```python
from build123d import *

# Parameters (mm, degrees)
SKETCH1_W                 = 270
SKETCH1_H                 = 130
SKETCH1_W_2               = 246
SKETCH1_H_2               = 106
BOSS_EXTRUDE1_DEPTH       = 12
SKETCH3_R                 = 2
CUT_EXTRUDE1_DEPTH        = 50.25
LPATTERN1_COUNT           = 2
LPATTERN1_PITCH           = 31
LPATTERN1_COPY_1_SKETCH_R = 2
LPATTERN1_COPY_1_DEPTH    = 50.25
LPATTERN2_COUNT           = 2
LPATTERN2_PITCH           = 161
MIRROR2_COPY_1_SKETCH_R   = 2
MIRROR2_COPY_1_DEPTH      = 50.25
MIRROR2_COPY_2_SKETCH_R   = 2
MIRROR2_COPY_2_DEPTH      = 50.25


with BuildPart() as part:
    # Sketch1 → Boss-Extrude1 (new body)
    with BuildSketch(Plane(origin=(0, 0, 0), x_dir=(1, 0, 0), z_dir=(0, 1, 0))):
        Rectangle(SKETCH1_W, SKETCH1_H)
        Rectangle(SKETCH1_W_2, SKETCH1_H_2, mode=Mode.SUBTRACT)
    extrude(amount=BOSS_EXTRUDE1_DEPTH)

    # Sketch3 → Cut-Extrude1 (cut)
    with BuildSketch(Plane(origin=(0, 12, 0), x_dir=(1, 0, 0), z_dir=(0, 1, 0))):
        with Locations((-65.5, -59)):
            Circle(SKETCH3_R)
    cut_extrude1 = extrude(amount=-CUT_EXTRUDE1_DEPTH, mode=Mode.SUBTRACT)

    # Mirror1: Cut-Extrude1 across plane
    add(cut_extrude1.mirror(Plane.XY), mode=Mode.SUBTRACT)

    # LPattern1: Cut-Extrude1 ×2
    with Locations(*[(i * LPATTERN1_PITCH, 0, 0) for i in range(1, LPATTERN1_COUNT)]):
        add(cut_extrude1, mode=Mode.SUBTRACT)

    # LPattern1 copy 1 sketch → LPattern1 copy 1 (cut)
    with BuildSketch(Plane(origin=(31, 12, 0), x_dir=(1, 0, 0), z_dir=(0, 1, 0))):
        with Locations((-65.5, 59)):
            Circle(LPATTERN1_COPY_1_SKETCH_R)
    extrude(amount=-LPATTERN1_COPY_1_DEPTH, mode=Mode.SUBTRACT)

    # LPattern2: Cut-Extrude1 ×2
    with Locations(*[(i * LPATTERN2_PITCH, 0, 0) for i in range(1, LPATTERN2_COUNT)]):
        add(cut_extrude1, mode=Mode.SUBTRACT)

    # Mirror2 copy 1 sketch → Mirror2 copy 1 (cut)
    with BuildSketch(Plane(origin=(161, 12, 0), x_dir=(1, 0, 0), z_dir=(0, 1, 0))):
        with Locations((-65.5, 59)):
            Circle(MIRROR2_COPY_1_SKETCH_R)
    extrude(amount=-MIRROR2_COPY_1_DEPTH, mode=Mode.SUBTRACT)

    # Mirror2 copy 2 sketch → Mirror2 copy 2 (cut)
    with BuildSketch(Plane(origin=(0, 12, 0), x_dir=(1, 0, 0), z_dir=(0, 1, 0))):
        with Locations((-65.5, 59)):
            Circle(MIRROR2_COPY_2_SKETCH_R)
    extrude(amount=-MIRROR2_COPY_2_DEPTH, mode=Mode.SUBTRACT)


solid = part.part
```
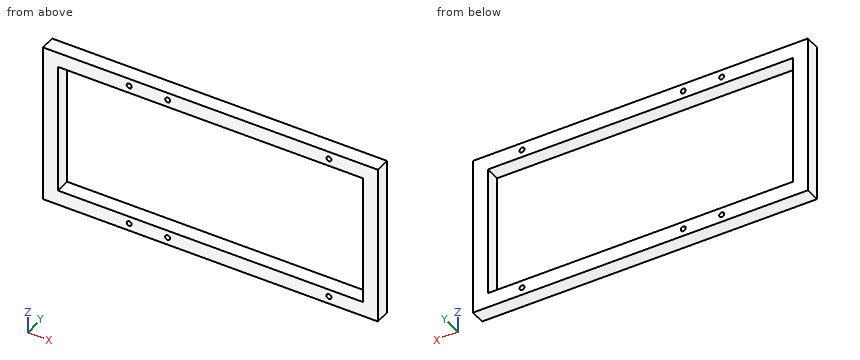
Design review of the part built by this model. Coordinates are the model's own, in mm. Give positions to 0.01 mm unless a question says otherwise; leave off trailing zeros. Order: outer loops, then holes, each group sorted by start corner. A loop starts at its lowest first (then second) coordinate and runs counter-clockwise, first axis right, second up. Notation, with made-up numbers: (16.25, -10) - (65.25, -10) arc R17 cw to (65.25, 8) - close; hole circle Ø10 at (-25.5, -28). An arc over 180 degrees is marked (long way). Use a Markdown table: item, result. Add a question column.
(1) Add section B-B on y = 6. Give the boundary of the cut face in (x, z).
(2) Wall thickness on probe 1 along X at (y, z) = (4, -59); probe 2 along Z at (x, y) = (-34.5, 5); probe 3 along Z at (x, y) = (120.5, 7): over which ranges is each line inside the solid? List them lowest first. Write a range as [from, to].
(3) Add section A-A on x = 39. Give the boundary of the cut face in (y, z).
(4) Add section C-C on z = -12.5. Give the boundary of the cut face in (x, y).
Report:
| question | item | result |
|---|---|---|
| 1 | outline | (-135, -65) - (135, -65) - (135, 65) - (-135, 65) - close; hole (-123, -53) - (123, -53) - (123, 53) - (-123, 53) - close; hole circle Ø4 at (-65.5, -59); hole circle Ø4 at (-65.5, 59); hole circle Ø4 at (-34.5, -59); hole circle Ø4 at (-34.5, 59); hole circle Ø4 at (95.5, -59); hole circle Ø4 at (95.5, 59) |
| 2 | probe 1 | x = [-135, -67.5], [-63.5, -36.5], [-32.5, 93.5], [97.5, 135] |
| 2 | probe 2 | z = [-65, -61], [-57, -53], [53, 57], [61, 65] |
| 2 | probe 3 | z = [-65, -53], [53, 65] |
| 3 | outline | (0, -65) - (12, -65) - (12, -53) - (0, -53) - close; (0, 53) - (12, 53) - (12, 65) - (0, 65) - close |
| 4 | outline | (-135, 0) - (-123, 0) - (-123, 12) - (-135, 12) - close; (123, 0) - (135, 0) - (135, 12) - (123, 12) - close |
